```python
from build123d import *

# Parameters (mm, degrees)
BOSS_EXTRUDE1_DEPTH = 35
SHELL1_T            = -3
SKETCH2_W           = 26
SKETCH2_H           = 26
CUT_EXTRUDE1_DEPTH  = 36
SKETCH3_R           = 4
CUT_EXTRUDE2_DEPTH  = 36


with BuildPart() as part:
    # Sketch1 → Boss-Extrude1 (new body)
    with BuildSketch(Plane(origin=(0, 0, 0), x_dir=(1, 0, 0), z_dir=(0, 1, 0))):
        Polygon((-325, -12.5), (-290, 22.5), (290, 22.5), (325, -12.5), align=None)
    extrude(amount=BOSS_EXTRUDE1_DEPTH)

    # Shell1
    shell1_openings = [part.faces().sort_by_distance(p)[0] for p in [
        (-307.5, 17.5, -5),
        (307.5, 17.5, -5),
    ]]
    offset(amount=SHELL1_T, openings=shell1_openings, kind=Kind.INTERSECTION)

    # Sketch2 → Cut-Extrude1 (cut, through all)
    with BuildSketch(Plane.XY.offset(12.5)):
        with Locations((0, 17.5)):
            Rectangle(SKETCH2_W, SKETCH2_H)
    extrude(amount=-CUT_EXTRUDE1_DEPTH, mode=Mode.SUBTRACT)

    # Sketch3 → Cut-Extrude2 (cut, through all)
    with BuildSketch(Plane(origin=(0, 35, 0), x_dir=(1, 0, 0), z_dir=(0, 1, 0))):
        with Locations((0, 5)):
            Circle(SKETCH3_R)
        with Locations((140, 5)):
            Circle(SKETCH3_R)
        with Locations((-140, 5)):
            Circle(SKETCH3_R)
    extrude(amount=-CUT_EXTRUDE2_DEPTH, mode=Mode.SUBTRACT)


solid = part.part
```
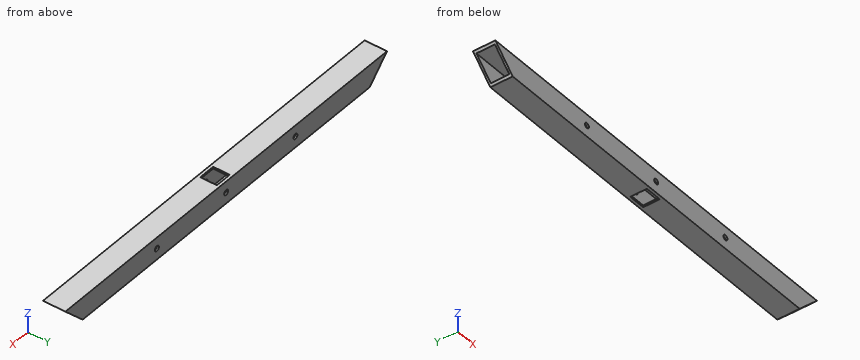
Design review of the part built by this model. Coordinates are the model's own, in mm. Round coordinates to 2 decimals unless told otherwise and drop trailing zeros. Write each loop counter-clockwise with the first axis right and the second up, starting at its lowest first coordinate (ties: lowest second). Pieces come first, ordered by that corner, then holes.
Item 1: We need section A-A on y = 12.5. Write out the cut boundary in (x, z), and give its area (3 significant figures).
Item 2: For probe 1 along Z at (x, y) = (177.5, 24); probe 2 along Y at (x, z) = (11, 2); probe 3 along Z at (x, y) = (0, 0.7), list the stretches that pass through material, from the lowest coordinate up.
Item 3: Clearance check with flat-ended pins moving along their axes: pin 1 Ø2.5 at (y, z) = (12, -20.5) entering from -X; pin 2 Ø1.5 at (y, z) = (22, 10.5) entering from +X; pin 3 Ø7 at (x, z) = (140, -5) entering from +Y; pin 4 Ø3.5 at (y, z) = (22, -21) entering from +X. State where each tip first meets the part, or that it passes through.
Item 4: We need section B-B on x = 38. Write out the cut boundary in (y, z).
Returned:
1. outline: (-325, 12.5) - (-322, 9.5) - (-13, 9.5) - (-13, 12.5) - close; (-293, -19.5) - (-290, -22.5) - (-13, -22.5) - (-13, -19.5) - close; (13, -22.5) - (290, -22.5) - (293, -19.5) - (13, -19.5) - close; (13, 9.5) - (322, 9.5) - (325, 12.5) - (13, 12.5) - close
1. area: 3,530 mm2
2. probe 1: z = -22.5 to -19.5, 9.5 to 12.5
2. probe 2: y = 0 to 3, 32 to 35
2. probe 3: z = -22.5 to -9, -1 to 12.5
3. pin 1: stops at x = -293
3. pin 2: stops at x = 323.75
3. pin 3: passes through
3. pin 4: stops at x = 293
4. outline: (0, -22.5) - (35, -22.5) - (35, 12.5) - (0, 12.5) - close; hole (3, -19.5) - (32, -19.5) - (32, 9.5) - (3, 9.5) - close
